The listing builds one solid part. Answer for the finished solid, in the listing's coordinates (mm). Round coordinates to 2 decimals unless told otherwise and drop trailing zeros. Loops run counter-clockwise (first coordinate to the right, second up) from the corner with the lowest first, then second, coordinate; pieces in that order, holes last. Notation, with made-up numbers: M 12,53 L 57,53 A12 ccw 57,60 Z; hole C 18,-37 d6. An arc over 180 degrees is marked long. Put each result on its own line as item: value. Start each with the question number.
(1) Straight lines are drawn through the part: line 1 (X direction, y = -1.7, z = 25.45); line 2 (X direction, y = -0.8, z = 25.95). For each, find the intervals that lie inside material, in ascending order.
(2) A flat-ended cylindrical pin translates along its axis: P1, Ø1, axis at y = -2.5, z = 26.5, coming from the -X side. Find the tip coordinate at first contact, or state that the pin passes through.
(3) Section A-A, the plane z = 25.05 is taken. Determine the outline of the cut face in (x, y) (3 decimals).
(4) Section B-B, the plane y = -2.55 is taken. Determine the outline of the cut face in (x, z).
```python
from build123d import *

# Parameters (mm, degrees)
F0_W        = 152.4
F0_H        = 3.175
F1_DEPTH    = 3.175
F2_T1_DEPTH = 23.6619672735
F3_T1_DEPTH = 35.0436157588


# Not quite as in the source:
# - a fillet or chamfer that OpenCascade refuses, or shapes differently, is made with other operations: its cross-section is extruded or revolved along the edge and cut away or added


with BuildPart() as f1:
    # F0 (on Front) → F1 (new body)
    with BuildSketch(Plane.XZ):
        with Locations((18.7120195478, 26.0135995823)):
            Rectangle(F0_W, F0_H)
    extrude(amount=F1_DEPTH)

    # F2: chamfer of 2.286 x 3.9594681461 on 1 edges, made by hand

    # F2_s2 → F2_t1 (cut)
    with BuildSketch(Plane.XY.offset(14.1826159455)):
        Polygon((-57.4879804522, 0.7844681461), (-55.2019804522, -3.175), (-57.4879804522, -3.175), align=None)
    extrude(amount=F2_T1_DEPTH, mode=Mode.SUBTRACT)

    # F3: chamfer of 3.556 x 6.1591726717 on 1 edges, made by hand

    # F3_s2 → F3_t1 (cut)
    with BuildSketch(Plane.XY.offset(8.4917917029)):
        Polygon((88.7528468761, -3.175), (94.9120195478, 0.381), (94.9120195478, -3.175), align=None)
    extrude(amount=F3_T1_DEPTH, mode=Mode.SUBTRACT)


solid = f1.part
```
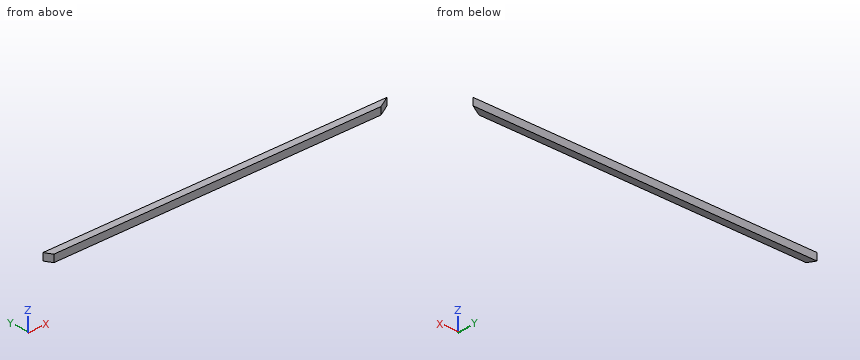
Recorded:
1. line 1: x = -56.05 to 91.31
1. line 2: x = -56.57 to 92.87
2. P1: stops at x = -55.88
3. outline: M -57.035,0 L -55.202,-3.175 L 88.753,-3.175 L 94.252,0 Z
4. outline: M -55.56,24.43 L 89.84,24.43 L 89.84,27.6 L -55.56,27.6 Z
